Here's how the part is built. I have some questions about the finished solid (model axes, mm). Face numbers are marked on the shaded views. A direction names the side the tool comes from. Round coordinates to 2 decimals unless told otherwise and drop trailing zeros. Write each loop counter-clockwise with the first axis right and the second up, starting at its lowest first coordinate (ties: lowest second). Pieces come first, ordered by that corner, then holes. Notation, with made-up numbers: (-11.5, 24.5) -> (29.5, 24.5) arc R24 cw to (29.5, 45.5) -> close; hole circle Ø7 at (-23, 81.25). An arc over 180 degrees is marked (long way). Answer in a Markdown table with one row per item.
from build123d import *

# Parameters (mm, degrees)
BOSS_EXTRUDE1_DEPTH = 17.5
BOSS_EXTRUDE2_START = 1
SKETCH2_W           = 0.5
SKETCH2_H           = 5
BOSS_EXTRUDE2_DEPTH = 37
SKETCH3_R           = 3
SKETCH3_R_2         = 1.65
CUT_EXTRUDE1_DEPTH  = 54.605037077
SKETCH4_W           = 35
SKETCH4_H           = 35
SKETCH4_R           = 15
BOSS_EXTRUDE3_DEPTH = 42
CUT_EXTRUDE2_DEPTH  = 67.697076398
SKETCH6_R           = 5
CUT_EXTRUDE3_DEPTH  = 73.301452268
SKETCH7_R           = 2.25
CUT_EXTRUDE4_DEPTH  = 73.3014524
CHAMFER1_SIZE       = 2
SKETCH8_W           = 7
SKETCH8_H           = 2.914047854
CUT_EXTRUDE5_DEPTH  = 42


with BuildPart() as part:
    # Sketch1 → Boss-Extrude1 (new, symmetric)
    with BuildSketch(Plane.XY):
        Polygon((0.5, -17.5), (15.5, -17.5), (15.5, 17.5), (18.5, 17.5), (18.5, -17.5), (60.5, -17.5), (60.5, -22.5), (0.5, -22.5), align=None)
    extrude(amount=BOSS_EXTRUDE1_DEPTH, both=True)

    # Sketch2 → Boss-Extrude2 (add)
    with BuildSketch(Plane.XY.offset(17.5).offset(BOSS_EXTRUDE2_START)):
        with Locations((44.45, -20)):
            Rectangle(SKETCH2_W, SKETCH2_H)
    extrude(amount=-BOSS_EXTRUDE2_DEPTH)

    # Sketch3 → Cut-Extrude1 (cut, through all)
    with BuildSketch(Plane.ZY.offset(-15.5)):
        Circle(SKETCH3_R)
        with Locations((-5.656854249, 5.656854249)):
            Circle(SKETCH3_R_2)
        with Locations((5.656854249, 5.656854249)):
            Circle(SKETCH3_R_2)
        with Locations((5.656854249, -5.656854249)):
            Circle(SKETCH3_R_2)
        with Locations((-5.656854249, -5.656854249)):
            Circle(SKETCH3_R_2)
    extrude(amount=-CUT_EXTRUDE1_DEPTH, mode=Mode.SUBTRACT)

    # Sketch4 → Boss-Extrude3 (add, through all)
    with BuildSketch(Plane(origin=(18.5, 0, 0), x_dir=(0, 0, -1), z_dir=(1, 0, 0))):
        Rectangle(SKETCH4_W, SKETCH4_H)
        with Locations(Location((0, 0, 0), (0, 0, 180))):
            Circle(SKETCH4_R, mode=Mode.SUBTRACT)
    extrude(amount=BOSS_EXTRUDE3_DEPTH)

    # Sketch5 → Cut-Extrude2 (cut, through all)
    with BuildSketch(Plane(origin=(60.5, 0, 0), x_dir=(0, 0, -1), z_dir=(1, 0, 0))):
        with BuildLine():
            Line((-17.5, 0), (-17.5, 18.5))
            Line((-17.5, 18.5), (17.5, 18.5))
            Line((17.5, 18.5), (17.5, 0))
            ThreePointArc((17.5, 0), (0, 17.5), (-17.5, 0))
        make_face()
    extrude(amount=-CUT_EXTRUDE2_DEPTH, mode=Mode.SUBTRACT)

    # Sketch6 → Cut-Extrude3 (cut, through all)
    with BuildSketch(Plane(origin=(0, -17.5, 0), x_dir=(1, 0, 0), z_dir=(0, 1, 0))):
        with Locations(Location((31.475, -10.5, 0), (0, 0, 90))):
            Circle(SKETCH6_R)
        with Locations(Location((31.475, 10.5, 0), (0, 0, 90))):
            Circle(SKETCH6_R)
    extrude(amount=CUT_EXTRUDE3_DEPTH, mode=Mode.SUBTRACT)

    # Sketch7 → Cut-Extrude4 (cut, through all)
    with BuildSketch(Plane(origin=(0, -17.5, 0), x_dir=(1, 0, 0), z_dir=(0, 1, 0))):
        with Locations(Location((8, 10.5, 0), (0, 0, 270))):
            Circle(SKETCH7_R)
        with Locations(Location((8, -10.5, 0), (0, 0, 270))):
            Circle(SKETCH7_R)
        with Locations(Location((31.475, -10.5, 0), (0, 0, 270))):
            Circle(SKETCH7_R)
        with Locations(Location((31.475, 10.5, 0), (0, 0, 270))):
            Circle(SKETCH7_R)
    extrude(amount=-CUT_EXTRUDE4_DEPTH, mode=Mode.SUBTRACT)

    # Chamfer1
    chamfer1_edges = [part.edges().sort_by_distance(p)[0] for p in [
        (31.475, -17.5, 8.25),
        (8, -17.5, -12.75),
        (31.475, -17.5, -12.75),
        (8, -17.5, 8.25),
    ]]
    chamfer(chamfer1_edges, length=CHAMFER1_SIZE)

    # Sketch8 → Cut-Extrude5 (cut)
    with BuildSketch(Plane(origin=(60.5, 0, 0), x_dir=(0, 0, -1), z_dir=(1, 0, 0))):
        with Locations((0, 16.042976073)):
            Rectangle(SKETCH8_W, SKETCH8_H)
    extrude(amount=-CUT_EXTRUDE5_DEPTH, mode=Mode.SUBTRACT)


solid = part.part
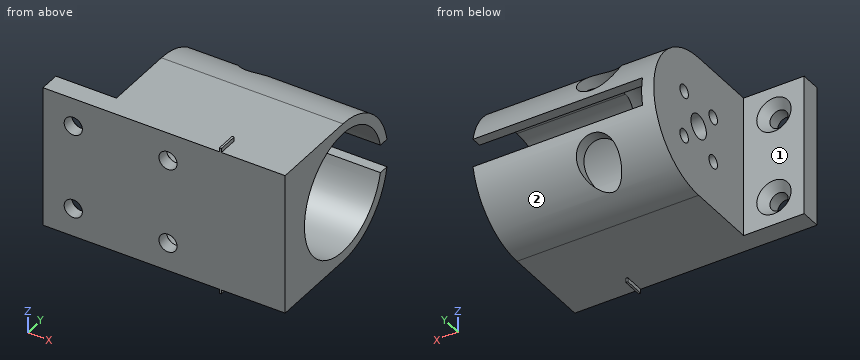
1) Which directions (+Z, -Z, +X, -X, +Y, -Y) give clear straight access to the entire face, cutting with the end or side of a thin tool? Please do the marked faces 1 and 2.
Response:
| item | result |
|---|---|
| face 1 | +Z, -Z, -X, +Y |
| face 2 | +X, -X, +Y |
2) For pin 1 (10.5 mm diameter, centred on y = 0.5, z = 7, fed in from -X); pin 2 (6 mm diameter, centred on x = 19, z = 7, fed in from +Y); pin 3 (18 mm diameter, centred on x = 34.5, y = -10, fed in from +Z), each with a flat end and sliding along its axis, tell me the tip position at first contact or that it passes through.
Response:
| item | result |
|---|---|
| pin 1 | stops at x = 15.5 |
| pin 2 | stops at y = 17.04 |
| pin 3 | stops at z = 17.5 |
3) I need wall thicknesses on line 1 (X direction, y = -21.5, z = -10.5) (3 decimals); line 2 (X direction, y = -9, z = -4.5); line 3 (X direction, y = -13, z = -14.5) (3 decimals). Which ranges of each line are inside material? Lowest first, please. Write a range as [from, to].
Response:
| item | result |
|---|---|
| line 1 | x = [0.5, 5.75], [10.25, 29.225], [33.725, 60.5] |
| line 2 | x = [15.5, 18.5] |
| line 3 | x = [15.5, 28.475], [34.475, 60.5] |
4) I want a section at B-B, the plane z = 10.5. Count the separate pieces of the cut face and the enclosed holes in it, and give its area (3 significant figures).
Response:
| item | result |
|---|---|
| separate pieces | 4 |
| enclosed holes | 0 |
| area | 664 mm^2 |
5) I want a section at D-D, the plane x = 41. List the corners of the cut face in (y, z) for me.
Response:
| item | result |
|---|---|
| outline | (-22.5, -17.5) -> (0, -17.5) arc R17.5 ccw to (17.15, -3.5) -> (14.59, -3.5) arc R15 cw (long way) to (14.59, 3.5) -> (17.15, 3.5) arc R17.5 ccw to (0, 17.5) -> (-22.5, 17.5) -> close |
6) I want a section at A-A, the plane z = 0. List the corners of the cut face in (x, y) for me, and give its area (3 significant figures).
Response:
| item | result |
|---|---|
| outline | (0.5, -22.5) -> (60.5, -22.5) -> (60.5, -15) -> (18.5, -15) -> (18.5, -3) -> (15.5, -3) -> (15.5, -17.5) -> (0.5, -17.5) -> close; (15.5, 3) -> (18.5, 3) -> (18.5, 17.5) -> (15.5, 17.5) -> close |
| area | 492 mm^2 |
7) I want a section at C-C, the plane x = 16.5. List the corners of the cut face in (y, z) for me.
Response:
| item | result |
|---|---|
| outline | (-22.5, -17.5) -> (0, -17.5) arc R17.5 ccw to (0, 17.5) -> (-22.5, 17.5) -> close; hole circle Ø3.3 at (-5.66, -5.66); hole circle Ø3.3 at (-5.66, 5.66); hole circle Ø6 at (0, 0); hole circle Ø3.3 at (5.66, -5.66); hole circle Ø3.3 at (5.66, 5.66) |
